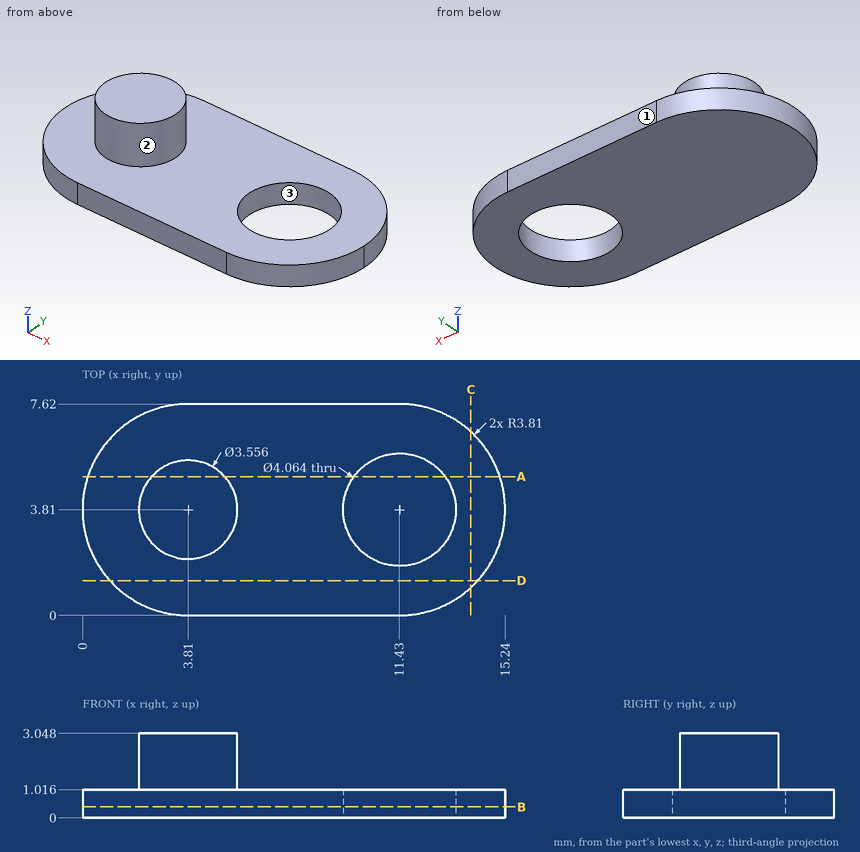
Print and shaded views of the part. All mm, measured from the part's lowest x, y and z. Round coordinates to 2 decimals unless told otherwise and drop trailing zeros. Order: outer loops, then holes, each group sorted by start corner. A loop starts at its lowest first (then second) coordinate and runs counter-clockwise, first axis right, second up.
Q1. Slice it at A-A (y = 5). Write the cut outline in (x, z).
Q2. Two-plate mould, pull along Y, no slides. Class the marked faces 1, 2 and 3: pulls with the +Y half, pulls with the -Y half, needs draft (parallel to the pull), parting line crosses it, or undercut.
Q3. Wall check: L1, parallel to X at y = 3.75, z = 0.7; L2, parallel to Y at x = 11.43, z = 0.65; L3, parallel to Z at x = 5, y = 6.5. Give the ranges that are in metal, low to high.
Q4. Slice it at D-D (y = 1.25). Write the cut outline in (x, z), and give its area (3 significant figures).
Q5. Drop a flat-ended pin along its axis: pin 1 (1 mm diameter, centred on y = 5, z = 2.5, fed in from +X). Give the stop position or say it passes through.
Q6. Slice it at B-B (z = 0.4). Write the cut outline in (x, y).
Q7. Slice it at C-C (x = 14). Write the cut outline in (y, z), and give its area (3 significant figures).
Results below:
1. outline: (0.19, 0) - (9.78, 0) - (9.78, 1.02) - (5.13, 1.02) - (5.13, 3.05) - (2.49, 3.05) - (2.49, 1.02) - (0.19, 1.02) - close; (13.08, 0) - (15.05, 0) - (15.05, 1.02) - (13.08, 1.02) - close
2. face 1: pulls with the +Y half
2. face 2: parting line crosses it
2. face 3: undercut
3. L1: x = 0 to 9.4, 13.46 to 15.24
3. L2: y = 0 to 1.78, 5.84 to 7.62
3. L3: z = 0 to 1.02
4. outline: (0.99, 0) - (14.25, 0) - (14.25, 1.02) - (0.99, 1.02) - close
4. area: 13.5 mm2
5. pin 1: stops at x = 5.45
6. outline: (3.81, 0) - (11.43, 0) arc R3.81 ccw to (15.24, 3.81) arc R3.81 ccw to (11.43, 7.62) - (3.81, 7.62) arc R3.81 ccw to start; hole circle Ø4.06 at (11.43, 3.81)
7. outline: (1, 0) - (6.62, 0) - (6.62, 1.02) - (1, 1.02) - close
7. area: 5.72 mm2
